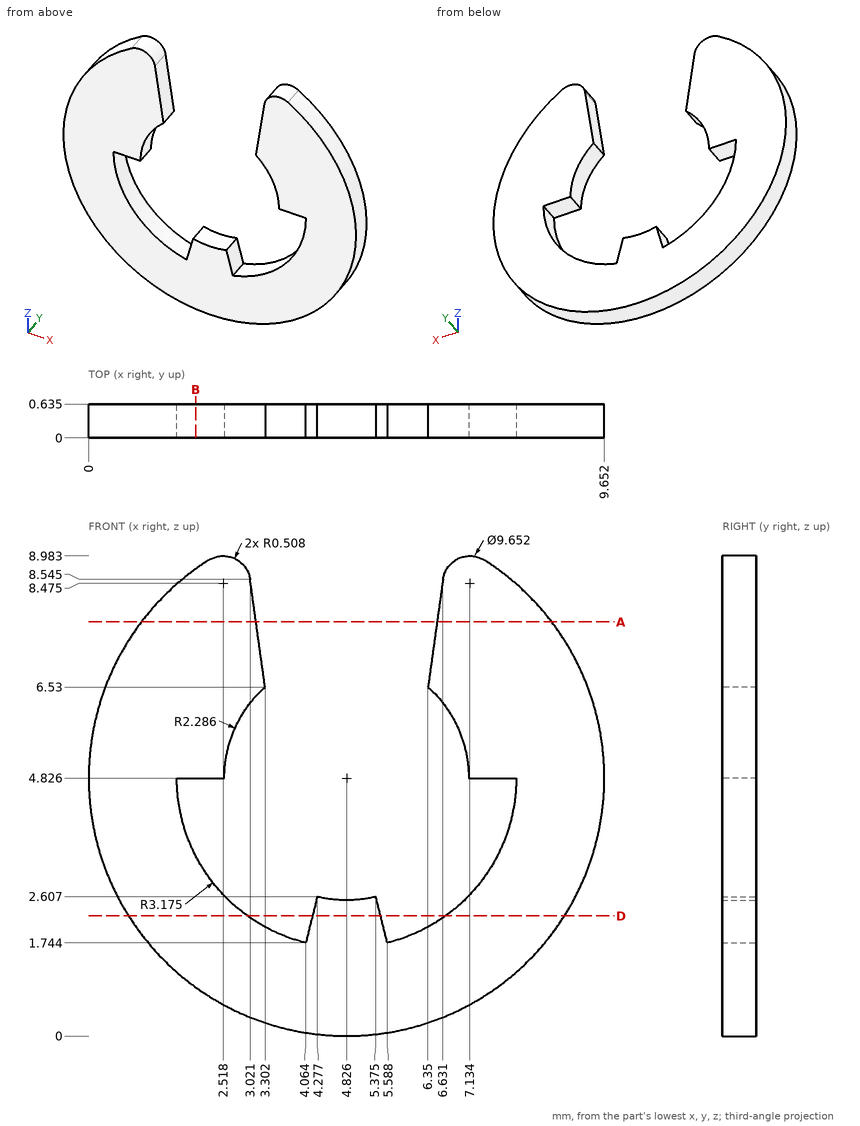
Here's the drawing with two shaded views (mm, measured from the low corner). I have some questions. Coordinates: 2 decimals unless noted, no trailing zeros. Write each loop counter-clockwise with the first axis right and the second up, starting at its lowest first coordinate (ties: lowest second). Pieces come first, ordered by that corner, then holes. Notation, with made-up numbers: (36.5, 9.25) - (72.5, 9.25) arc R4 cw to (72.5, 15.25) - close; hole circle Ø8 at (-36.5, 73). An arc over 180 degrees is marked (long way). Return JSON: item names as keys, results as strings.
Q1. If we section it at B-B (x = 2): Please give me the cut outline in (y, z) (1 decimal).
Computed values:
{"outline": "(0, 0.9) - (0.6, 0.9) - (0.6, 3.4) - (0, 3.4) - close; (0, 4.8) - (0.6, 4.8) - (0.6, 8.7) - (0, 8.7) - close"}
Q2. I'm going to push a flat-ended pin straight in: pin 1 Ø5 at (x, z) = (4, 4.5) entering from +Y (3 decimals). Where does the tip first touch, or does it pass through?
Computed values:
{"pin 1": "stops at y = 0.635"}
Q3. If we section it at A-A (z = 7.75): Please give me the cut outline in (x, y) (1 decimal).
Computed values:
{"outline": "(1, 0) - (3.1, 0) - (3.1, 0.6) - (1, 0.6) - close; (6.5, 0) - (8.7, 0) - (8.7, 0.6) - (6.5, 0.6) - close"}
Q4. If we section it at D-D (z = 2.25): Please give me the cut outline in (x, y) (1 decimal).
Computed values:
{"outline": "(0.7, 0) - (3, 0) - (3, 0.6) - (0.7, 0.6) - close; (4.2, 0) - (5.5, 0) - (5.5, 0.6) - (4.2, 0.6) - close; (6.7, 0) - (8.9, 0) - (8.9, 0.6) - (6.7, 0.6) - close"}
Q5. Please list where these lines run through material, in increasing order: L1, parallel to X at y = 0.2, z = 7.75 (1 decimal); L2, parallel to X at y = 0.35, z = 3.75; L3, parallel to Z at x = 7.75, y = 0.55 (1 decimal). Write a range as from..to.
Computed values:
{"L1": "x = 1..3.1, 6.5..8.7", "L2": "x = 0.12..1.84, 7.81..9.53", "L3": "z = 1..3.6, 4.8..8.7"}
